Work out the finished part from the listing and answer in its coordinate system (mm). Give positions to 0.01 mm unless a question says otherwise; leave off trailing zeros. Write each loop counter-clockwise with the first axis right and the second up, starting at its lowest first coordinate (ties: lowest second). Pieces come first, ordered by that corner, then holes. Notation, with made-up numbers: (27, 53) -> (75, 53) arc R18 cw to (75, 61) -> close; hole circle Ø11 at (48, 49). An arc over 180 degrees is marked (long way). Use a Markdown table: item, result. Add a question column.
Q1. Each of these flat-tipped pins is pushed along its axis until it touches: pin 1 Ø2.5 at (x, z) = (25.4, -63.5) entering from +Y; pin 2 Ø4 at (x, z) = (-63.5, 63.5) entering from +Y. Where does it stop, or does it pass through?
Q2. Section B-B, the plane y = 0.75 is taken. State how many separate pieces and enclosed holes the cut face has, plus the area to 3 significant figures.
Q3. Consider line 1 (X direction, y = 1, z = -63.5) (3 decimals); line 2 (X direction, y = 0, z = 0) (1 decimal); line 3 (Z direction, x = 65, y = -0.5). Determine where each line is inside the solid, lowest interval first.
Q4. Section C-C, the plane z = 0 is taken. Give the vertices of the cut face in (x, y) (1 decimal).
Q5. Section D-D, the plane x = -63.5 is taken. Give the vertices of the cut face in (y, z) (3 decimals).
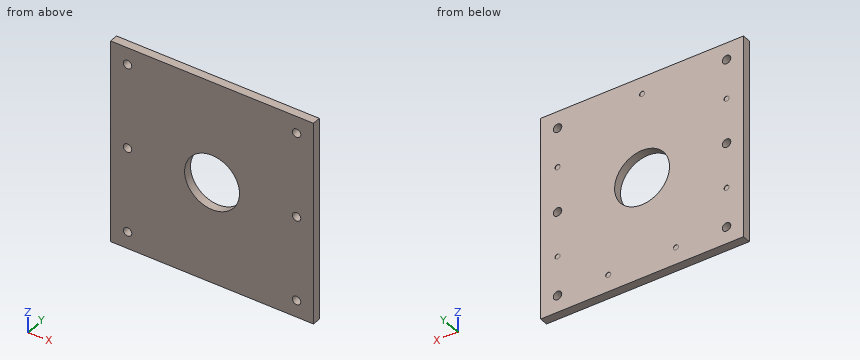
from build123d import *

# Parameters (mm, degrees)
SKETCH3_W           = 152.4
SKETCH3_H           = 6.35
BOSS_EXTRUDE1_DEPTH = 76.2
SKETCH4_R           = 3.175
CUT_EXTRUDE1_DEPTH  = 108.95
SKETCH5_R           = 1.905
SKETCH5_R_2         = 3.175
CUT_EXTRUDE2_DEPTH  = 0.254
SKETCH6_R           = 20.6375
CUT_EXTRUDE3_DEPTH  = 108.95


with BuildPart() as part:
    # Sketch3 → Boss-Extrude1 (new, symmetric)
    with BuildSketch(Plane.XY):
        Rectangle(SKETCH3_W, SKETCH3_H)
    extrude(amount=BOSS_EXTRUDE1_DEPTH, both=True)

    # Sketch4 → Cut-Extrude1 (cut, through all)
    with BuildSketch(Plane(origin=(0, 3.175, 0), x_dir=(1, 0, 0), z_dir=(0, 1, 0))):
        with Locations(Location((-63.5, 63.5, 0), (0, 0, 270))):
            Circle(SKETCH4_R)
        with Locations(Location((63.5, 63.5, 0), (0, 0, 270))):
            Circle(SKETCH4_R)
        with Locations(Location((63.5, 0, 0), (0, 0, 270))):
            Circle(SKETCH4_R)
        with Locations(Location((63.5, -63.5, 0), (0, 0, 270))):
            Circle(SKETCH4_R)
        with Locations(Location((-63.5, -63.5, 0), (0, 0, 270))):
            Circle(SKETCH4_R)
        with Locations(Location((-63.5, 0, 0), (0, 0, 270))):
            Circle(SKETCH4_R)
    extrude(amount=-CUT_EXTRUDE1_DEPTH, mode=Mode.SUBTRACT)

    # Sketch5 → Cut-Extrude2 (cut)
    with BuildSketch(Plane(origin=(0, 3.175, 0), x_dir=(1, 0, 0), z_dir=(0, 1, 0))):
        with Locations(Location((-25.4, 63.5, 0), (0, 0, 270))):
            Circle(SKETCH5_R)
        with Locations(Location((25.4, 63.5, 0), (0, 0, 270))):
            Circle(SKETCH5_R)
        with Locations(Location((63.5, 33.866666667, 0), (0, 0, 270))):
            Circle(SKETCH5_R)
        with Locations(Location((63.5, -33.866666667, 0), (0, 0, 270))):
            Circle(SKETCH5_R)
        with Locations(Location((0, -63.5, 0), (0, 0, 270))):
            Circle(SKETCH5_R)
        with Locations(Location((-63.5, -33.866666667, 0), (0, 0, 270))):
            Circle(SKETCH5_R)
        with Locations(Location((-63.5, 33.866666667, 0), (0, 0, 270))):
            Circle(SKETCH5_R)
        with Locations(Location((63.5, -63.5, 0), (0, 0, 270))):
            Circle(SKETCH5_R_2)
        with Locations(Location((-63.5, 63.5, 0), (0, 0, 270))):
            Circle(SKETCH5_R_2)
    extrude(amount=-CUT_EXTRUDE2_DEPTH, mode=Mode.SUBTRACT)

    # Sketch6 → Cut-Extrude3 (cut, through all)
    with BuildSketch(Plane(origin=(0, 3.175, 0), x_dir=(1, 0, 0), z_dir=(0, 1, 0))):
        with Locations(Location((0, 0, 0), (0, 0, 270))):
            Circle(SKETCH6_R)
    extrude(amount=-CUT_EXTRUDE3_DEPTH, mode=Mode.SUBTRACT)


solid = part.part
Result set:
| question | item | result |
|---|---|---|
| 1 | pin 1 | stops at y = 2.92 |
| 1 | pin 2 | passes through |
| 2 | separate pieces | 1 |
| 2 | enclosed holes | 7 |
| 2 | area | 21,700 mm2 |
| 3 | line 1 | x = -76.2 to -66.675, -60.325 to 60.325, 66.675 to 76.2 |
| 3 | line 2 | x = -76.2 to -66.7, -60.3 to -20.6, 20.6 to 60.3, 66.7 to 76.2 |
| 3 | line 3 | z = -76.2 to -66.3, -60.7 to -2.8, 2.8 to 60.7, 66.3 to 76.2 |
| 4 | outline | (-76.2, -3.2) -> (-66.7, -3.2) -> (-66.7, 3.2) -> (-76.2, 3.2) -> close; (-60.3, -3.2) -> (-20.6, -3.2) -> (-20.6, 3.2) -> (-60.3, 3.2) -> close; (20.6, -3.2) -> (60.3, -3.2) -> (60.3, 3.2) -> (20.6, 3.2) -> close; (66.7, -3.2) -> (76.2, -3.2) -> (76.2, 3.2) -> (66.7, 3.2) -> close |
| 5 | outline | (-3.175, -76.2) -> (3.175, -76.2) -> (3.175, -66.675) -> (-3.175, -66.675) -> close; (-3.175, -60.325) -> (3.175, -60.325) -> (3.175, -35.772) -> (2.921, -35.772) -> (2.921, -31.962) -> (3.175, -31.962) -> (3.175, -3.175) -> (-3.175, -3.175) -> close; (-3.175, 3.175) -> (3.175, 3.175) -> (3.175, 31.962) -> (2.921, 31.962) -> (2.921, 35.772) -> (3.175, 35.772) -> (3.175, 60.325) -> (-3.175, 60.325) -> close; (-3.175, 66.675) -> (3.175, 66.675) -> (3.175, 76.2) -> (-3.175, 76.2) -> close |
